For this review, take the finished solid that the model builds, in its own axes (mm). Face numbers are marked on the shaded views. A direction names the side the tool comes from. Coordinates: 2 decimals unless noted, no trailing zeros. Loops run counter-clockwise (first coordinate to the right, second up) from the corner with the lowest first, then second, coordinate; pieces in that order, holes last. Notation, with made-up numbers: (6.25, 63.5) -> (25.25, 63.5) arc R20 ccw to (25.25, 94.5) -> close; hole circle Ø3 at (59.5, 79). An arc over 180 degrees is marked (long way). One line per item, written item: value.
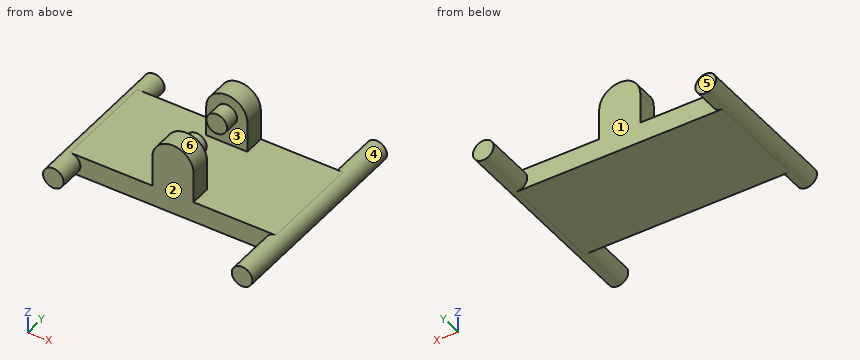
Autodesk Inventor part; units mm, degrees
ref_plane "YZ Plane" through (0, 0, 0) normal (1, 0, 0) x (0, 1, 0)
ref_plane "XZ Plane" through (0, 0, 0) normal (0, 1, 0) x (-1, 0, 0)
ref_plane "XY Plane" through (0, 0, 0) normal (0, 0, 1) x (1, 0, 0)
sketch "Sketch1" plane through (0, 0, 0) normal (0, 0, 1) x (1, 0, 0)
  line L0 (-50, 25) -> (50, 25)
  line L1 (50, 25) -> (50, -25)
  line L2 (50, -25) -> (-50, -25)
  line L3 (-50, -25) -> (-50, 25)
  point P0 (0, 0)
  dimension "d0" = 100
  dimension "d1" = 50
  dimension "d2" = 25
  dimension "d3" = 50
extrude "Extrusion1" add sketch "Sketch1" along normal mid plane 10
sketch "Sketch3" plane through (0, 0, 0) normal (0, 1, 0) x (-1, 0, 0)
  line L0 (50, -5) -> (50, 5)
  circle A0 centre (50, 0) radius 5
  line L1 (-50, -5) -> (-50, 5)
  point P0 (0, 0)
extrude "Extrusion2" add sketch "Sketch3" along normal mid plane 75
sketch "Sketch4" plane through (0, 0, 0) normal (0, 1, 0) x (-1, 0, 0)
  line L0 (-50, -5) -> (-50, 5)
  circle A0 centre (-50, 0) radius 5
  point P0 (0, 0)
extrude "Extrusion3" add sketch "Sketch4" along normal mid plane 100
sketch "Sketch8" plane through (-50, 25, 0) normal (0, 1, 0) x (1, 0, 0)
  line L0 (60, 0) -> (40, 0)
  line L1 (40, 0) -> (40, -20)
  line L2 (40, -20) -> (60, -20)
  line L3 (60, -20) -> (60, 0)
  arc A0 (40, -20) -> (60, -20) centre (50, -20) ccw
  point P0 (50, 0)
  dimension "d16" = 20
  dimension "d17" = 20
  dimension "d18" = 10
extrude "Extrusion6" add sketch "Sketch8" against normal blind 10
mirror "Mirror1" about plane through (0, 0, 0) normal (0, 1, 0) of "Extrusion6"
sketch "Sketch9" plane through (-50, 15, 0) normal (0, -1, 0) x (1, 0, 0)
  arc A0 (60, 20) -> (40, 20) centre (50, 20) ccw
  circle A1 centre (50, 20) radius 5
  point P0 (50, 0)
  dimension "d21" = 10
extrude "Extrusion7" add sketch "Sketch9" along normal blind 7.5
mirror "Mirror2" about plane through (0, 0, 0) normal (0, 1, 0) of "Extrusion7"
properties part number "enEffector" material "Stainless Steel"
1. Take a section at D-D, the plane y = 1.5. Give the boundary of the cut face in (x, z).
Return value:
outline: (-50, -5) -> (50, -5) arc R5 ccw to (50, 5) -> (-50, 5) arc R5 ccw to start
2. The part is to be moulded in two halves that separate along Y. For the marked faces 1, 2 and 3, say which applies: pulls with the +Y half, pulls with the -Y half, needs draft (parallel to the pull), parting line crosses it, or undercut.
Return value:
face 1: pulls with the +Y half
face 2: pulls with the -Y half
face 3: undercut
3. Insertion check: pin 1 Ø2 at (x, z) = (-4, 17) entering from -Y; pin 2 Ø11 at (y, z) = (-20, 11) entering from +X; pin 3 Ø12 at (x, z) = (14.5, 11.5) entering from +Y. Each pin has a flat end and moves straight along its axis. Give the tip position at first contact, or say it passes through.
Return value:
pin 1: stops at y = -25
pin 2: stops at x = 10
pin 3: stops at y = 25
4. For the marked faces 4, 5 and 6, list the 3-axis set-ups (+Z, -Z, +X, -X, +Y, -Y) from which the entire face can be reached by the end or side of a thin tool; tool diameter is ignored.
Return value:
face 4: none
face 5: +Z, -Z, -X, +Y
face 6: +Z, +Y, -Y
5. Take a section at B-B, the plane z = 0. Give the boundary of the cut face in (x, y).
Return value:
outline: (-55, -37.5) -> (-45, -37.5) -> (-45, -25) -> (45, -25) -> (45, -50) -> (55, -50) -> (55, 50) -> (45, 50) -> (45, 25) -> (-45, 25) -> (-45, 37.5) -> (-55, 37.5) -> close
6. To check wall thickness, follow probe 1 along Y at (x, z) = (-6.5, 9); probe 2 along X at (y, z) = (-11.5, -0.5); probe 3 along Y at (x, z) = (6.5, 0.5). State the ranges of each line that lie inside material, in increasing order. Write a range as from..to.
Return value:
probe 1: y = -25..-15, 15..25
probe 2: x = -54.97..54.97
probe 3: y = -25..25
7. Take a section at C-C, the plane x = 0. Give the boundary of the cut face in (y, z).
Return value:
outline: (-25, -5) -> (25, -5) -> (25, 30) -> (15, 30) -> (15, 25) -> (7.5, 25) -> (7.5, 15) -> (15, 15) -> (15, 5) -> (-15, 5) -> (-15, 15) -> (-7.5, 15) -> (-7.5, 25) -> (-15, 25) -> (-15, 30) -> (-25, 30) -> close
8. Take a section at A-A, the plane y = -11. Give the boundary of the cut face in (x, z), and give its area (3 significant figures).
Return value:
outline: (-50, -5) -> (50, -5) arc R5 ccw to (50, 5) -> (-50, 5) arc R5 ccw to start; circle Ø10 at (0, 20)
area: 1,160 mm2
